The listing builds one solid part. Answer for the finished solid, in the listing's coordinates (mm). A direction names the side the tool comes from. Round coordinates to 2 decimals unless told otherwise and drop trailing zeros. Order: outer loops, then holes, each group sorted by start corner. A loop starts at its lowest first (then second) coordinate and runs counter-clockwise, first axis right, second up. Notation, with made-up numbers: (-15.75, 36.5) - (-6.75, 36.5) arc R14 cw to (-6.75, 52.5) - close; hole circle Ø2 at (-8.75, 16.25). An arc over 180 degrees is marked (long way). One line per item, written item: value. Start each with the question number.
1. Section B-B, the plane y = -0.9 is taken. Count the separate pieces of the cut face and the enclosed holes in it, then the cut area to 3 significant figures.
2. Section C-C, the plane z = 165.1 is taken. Give the vertices of the cut face in (x, y) (3 decimals).
3. Straight lines are drawn through the part: line 1 (X direction, y = -2.05, z = 57.15) (3 decimals); line 2 (Z direction, x = 7.5, y = -2.05); line 3 (X direction, y = -0.7, z = 6.35) (3 decimals). For each, find the intervals that lie inside material, in ascending order.
4. Section D-D, the plane z = 61.5 is taken. Give the vertices of the cut face in (x, y) (3 decimals), then the cut area to 3 significant figures.
5. Section A-A, the plane z = 6.35 is taken. Give the vertices of the cut face in (x, y) (3 decimals).
6. A tool of negligible diameter and unlimited length cuts with its end or side. For faces 1 (the cylindrical face through (4.875, -1.565, 38.725)), 2 (the flat face through (0, -2, 36)), from which of +Z, -Z, +X, -X, +Y, -Y can it reach the whole face along a straight path? Write none if from no direction.
7. A flat-ended cylindrical pin translates along its axis: P1, Ø4, axis at x = -2.96, z = 100.38, coming from the +Y side. Find the tip coordinate at first contact, or state that the pin passes through.
8. For a pull along X with two mould halves and no side action, classify faces 3 (the cylindrical face through (-41.881, -1.565, 163.074)), 4 (the flat face through (-27.4, -1.57, 130.01)), 5 (the flat face through (15.875, -2, 35)) as released by +X, released by -X, zero draft, split by the parting line, or undercut.
from build123d import *

# Parameters (mm, degrees)
BASE_FLANGE1_DEPTH     = 3.175
SKETCH6_R              = 2.5527
CUT_EXTRUDE1_DEPTH     = 179.996051516
FILLET1_R              = 3.175
FILLET2_R              = 50.8
F_10_CLEARANCE_HOLE1_D = 5.1054


# Sheet-metal steps are written as plain solids
with BuildPart() as part:
    # Sketch1 → Base-Flange1 (new body)
    with BuildSketch(Plane(origin=(0, 0, 0), x_dir=(1, 0, 0), z_dir=(0, 1, 0))):
        Polygon((0, -82.55), (-51.326438931, -171.45), (-36.661742094, -171.45), (15.875, -80.45369343), (15.875, 0), (0, 0), align=None)
    extrude(amount=-BASE_FLANGE1_DEPTH)

    # Sketch6 → Cut-Extrude1 (cut, through all)
    with BuildSketch(Plane(origin=(0, 0, 0), x_dir=(1, 0, 0), z_dir=(0, 1, 0))):
        with Locations(Location((-40.327916303, -165.1, 0), (0, 0, 270))):
            Circle(SKETCH6_R)
        with Locations(Location((-14.927916303, -121.105909488, 0), (0, 0, 270))):
            Circle(SKETCH6_R)
        with Locations(Location((11.1125, -6.35, 0), (0, 0, 270))):
            Circle(SKETCH6_R)
        with Locations(Location((4.7625, -41.275, 0), (0, 0, 270))):
            Circle(SKETCH6_R)
        with Locations(Location((11.1125, -76.2, 0), (0, 0, 270))):
            Circle(SKETCH6_R)
    extrude(amount=-CUT_EXTRUDE1_DEPTH, mode=Mode.SUBTRACT)

    # Fillet1
    fillet1_edges = [part.edges().sort_by_distance(p)[0] for p in [
        (-36.661742094, -1.5875, 171.45),
        (-51.326438931, -1.5875, 171.45),
        (0, -1.5875, 0),
        (15.875, -1.5875, 0),
    ]]
    fillet(fillet1_edges, radius=FILLET1_R)

    # Fillet2
    fillet2_edges = [part.edges().sort_by_distance(p)[0] for p in [
        (0, -1.5875, 82.55),
        (15.875, -1.5875, 80.45369343),
    ]]
    fillet(fillet2_edges, radius=FILLET2_R)

    # #10 Clearance Hole1 (through all)
    with Locations(Plane(origin=(0, 0, 0), x_dir=(1, 0, 0), z_dir=(0, 1, 0))):
        with Locations((7.9375, -22.225), (7.9375, -57.15), (-2.964677617, -100.384972261), (-29.952177617, -147.12869343)):
            Hole(F_10_CLEARANCE_HOLE1_D / 2)


solid = part.part
Answer list:
1. separate pieces: 1
1. enclosed holes: 9
1. area: 2,420 mm²
2. outline: (-47.66, -3.175) - (-42.881, -3.175) - (-42.881, 0) - (-47.66, 0) - close; (-37.775, -3.175) - (-32.996, -3.175) - (-32.996, 0) - (-37.775, 0) - close
3. line 1: x = 0 to 5.385, 10.49 to 15.875
3. line 2: z = 0 to 19.71, 24.74 to 54.64, 59.66 to 94.96
3. line 3: x = 0 to 8.56, 13.665 to 15.875
4. outline: (0, -3.175) - (15.875, -3.175) - (15.875, 0) - (0, 0) - close
4. area: 50.4 mm²
5. outline: (0, -3.175) - (8.56, -3.175) - (8.56, 0) - (0, 0) - close; (13.665, -3.175) - (15.875, -3.175) - (15.875, 0) - (13.665, 0) - close
6. face 1: +Y, -Y
6. face 2: -Z, -X, +Y, -Y
7. P1: passes through
8. face 3: undercut
8. face 4: released by -X
8. face 5: released by +X
